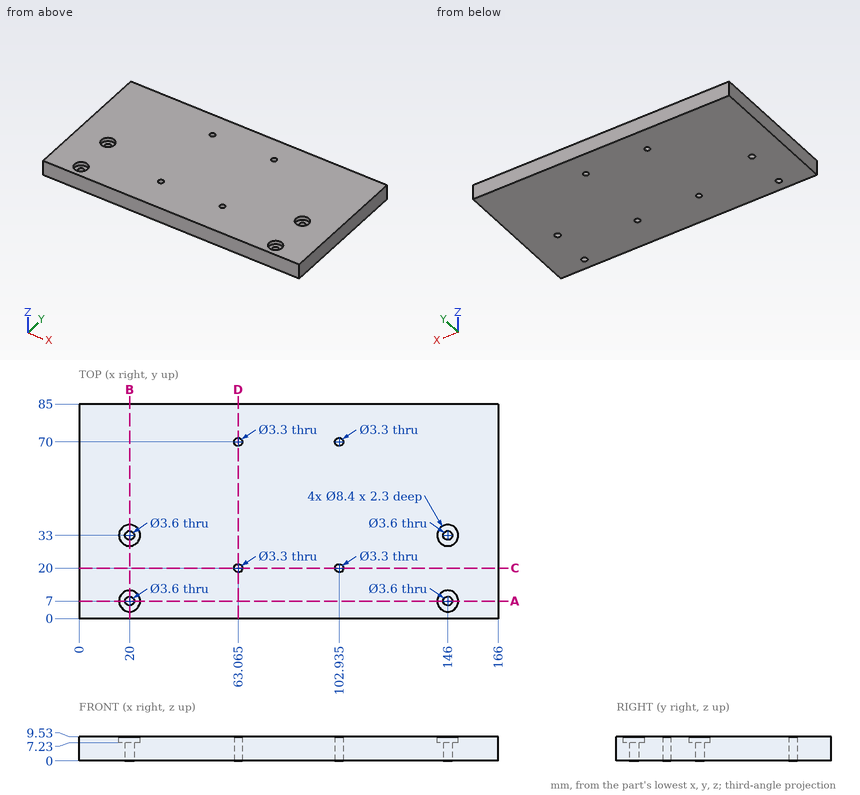
Geometry check sheet. Reference: drawing and pictorial views, mm from the part's lowest x, y, z. Round coordinates to 2 decimals unless told otherwise and drop trailing zeros. Loops run counter-clockwise (first coordinate to the right, second up) from the corner with the lowest first, then second, coordinate; pieces in that order, holes last. Notation, with made-up numbers: (38, 30) -> (61, 30) arc R15 ccw to (61, 35) -> close; hole circle Ø7 at (49, 83.5). An arc over 180 degrees is marked (long way). Use a Markdown table: item, result.
(1) Sectioned sample at A-A (y = 7). Enter the section's corners in (x, z), then the cut area to 3 significant figures.
Calculated:
| item | result |
|---|---|
| outline | (0, 0) -> (18.2, 0) -> (18.2, 7.23) -> (15.8, 7.23) -> (15.8, 9.53) -> (0, 9.53) -> close; (21.8, 0) -> (144.2, 0) -> (144.2, 7.23) -> (141.8, 7.23) -> (141.8, 9.53) -> (24.2, 9.53) -> (24.2, 7.23) -> (21.8, 7.23) -> close; (147.8, 0) -> (166, 0) -> (166, 9.53) -> (150.2, 9.53) -> (150.2, 7.23) -> (147.8, 7.23) -> close |
| area | 1,490 mm² |
(2) Sectioned sample at C-C (y = 20). Enter the section's corners in (x, z) (3 decimals).
Calculated:
| item | result |
|---|---|
| outline | (0, 0) -> (61.415, 0) -> (61.415, 9.53) -> (0, 9.53) -> close; (64.715, 0) -> (101.285, 0) -> (101.285, 9.53) -> (64.715, 9.53) -> close; (104.585, 0) -> (166, 0) -> (166, 9.53) -> (104.585, 9.53) -> close |
(3) Scan lines: probe 1 along Y at (x, z) = (146, 3.25); probe 2 along Y at (x, z) = (146, 7.8); probe 3 along X at (y, z) = (70, 7) (3 decimals). Record each from-to range of solid material in increasing order.
Calculated:
| item | result |
|---|---|
| probe 1 | 0 to 5.2, 8.8 to 31.2, 34.8 to 85 |
| probe 2 | 0 to 2.8, 11.2 to 28.8, 37.2 to 85 |
| probe 3 | 0 to 61.415, 64.715 to 101.285, 104.585 to 166 |
(4) Sectioned sample at D-D (x = 63). Enter the section's corners in (y, z).
Calculated:
| item | result |
|---|---|
| outline | (0, 0) -> (18.35, 0) -> (18.35, 9.53) -> (0, 9.53) -> close; (21.65, 0) -> (68.35, 0) -> (68.35, 9.53) -> (21.65, 9.53) -> close; (71.65, 0) -> (85, 0) -> (85, 9.53) -> (71.65, 9.53) -> close |
(5) Go/stop test with a flat-tipped pin: P1, Ø5, axis at x = 146, y = 33, coming from the +Z side. Record where the tip stops, or that it passes through.
Calculated:
| item | result |
|---|---|
| P1 | z = 7.23 |
(6) Sectioned sample at B-B (x = 20). Enter the section's corners in (y, z), then the cut area to 3 significant figures.
Calculated:
| item | result |
|---|---|
| outline | (0, 0) -> (5.2, 0) -> (5.2, 7.23) -> (2.8, 7.23) -> (2.8, 9.53) -> (0, 9.53) -> close; (8.8, 0) -> (31.2, 0) -> (31.2, 7.23) -> (28.8, 7.23) -> (28.8, 9.53) -> (11.2, 9.53) -> (11.2, 7.23) -> (8.8, 7.23) -> close; (34.8, 0) -> (85, 0) -> (85, 9.53) -> (37.2, 9.53) -> (37.2, 7.23) -> (34.8, 7.23) -> close |
| area | 719 mm² |
